Answer from the drawing. Dimensions are ordinates in mm from the lowest x, y and z of the part. Give positions to 0.01 mm unless a question says otherwise; leave off trailing zeros. Order: outer loops, then holes, each group sorted by start corner. A loop starts at its lowest first (then second) coordinate and runs counter-clockwise, first axis right, second up. Notation, with made-up numbers: (85.5, 35) - (110.5, 35) arc R11 ccw to (110.5, 47) - close; hole circle Ø11 at (0, 5.5). An arc over 180 degrees is marked (long way). Use a Markdown table: item, result. Add a question column.
1) Find section A-A, the plane z = 0.45. Determine the outline of the cut face in (x, y), plus the area to 3 significant figures.
2) Find section C-C, the plane y = 2.5. Determine the outline of the cut face in (x, z).
3) Find section B-B, the plane x = 26. Determine the outline of the cut face in (y, z), plus the area to 3 significant figures.
4) Straight lines are drawn through the part: line 1 (X direction, y = 4, z = 0.2); line 2 (Y direction, x = 27, z = 0.6); line 3 (Y direction, x = 9.5, z = 0.2). For each, find the intervals that lie inside material, in ascending order.
5) A flat-ended cylindrical pin translates along its axis: pin 1 (0.8 mm diameter, centred on x = 16.5, z = 1, fed in from -Y). Find the tip coordinate at first contact, or state that the pin passes through.
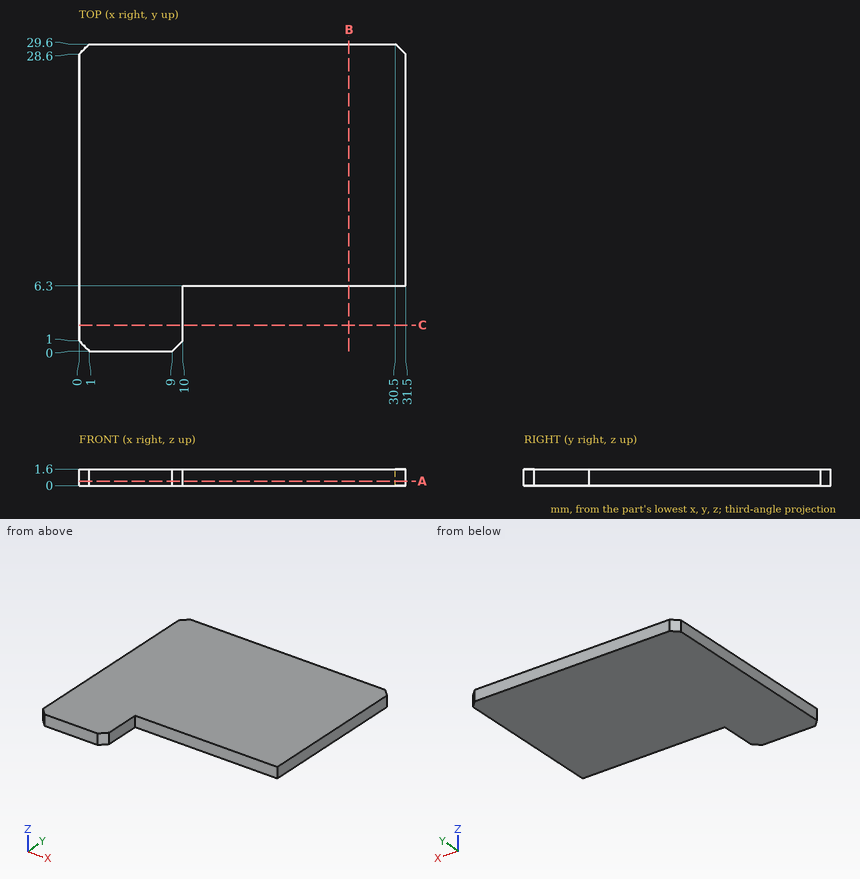
The answers:
| question | item | result |
|---|---|---|
| 1 | outline | (0, 1) - (1, 0) - (9, 0) - (10, 1) - (10, 6.3) - (31.5, 6.3) - (31.5, 28.6) - (30.5, 29.6) - (1, 29.6) - (0, 28.6) - close |
| 1 | area | 795 mm2 |
| 2 | outline | (0, 0) - (10, 0) - (10, 1.6) - (0, 1.6) - close |
| 3 | outline | (6.3, 0) - (29.6, 0) - (29.6, 1.6) - (6.3, 1.6) - close |
| 3 | area | 37.3 mm2 |
| 4 | line 1 | 0 to 10 |
| 4 | line 2 | 6.3 to 29.6 |
| 4 | line 3 | 0.5 to 29.6 |
| 5 | pin 1 | y = 6.3 |
